Autodesk Inventor part; units mm, degrees
ref_plane "YZ Plane" through (0, 0, 0) normal (1, 0, 0) x (0, 1, 0)
ref_plane "XZ Plane" through (0, 0, 0) normal (0, 1, 0) x (-1, 0, 0)
ref_plane "XY Plane" through (0, 0, 0) normal (0, 0, 1) x (1, 0, 0)
sketch "Sketch1" plane through (0, 0, 0) normal (0, 0, 1) x (1, 0, 0)
  line L0 (-205, -150) -> (205, -150)
  line L1 (205, -150) -> (205, 150)
  line L2 (205, 150) -> (-205, 150)
  line L3 (-205, 150) -> (-205, -150)
  line L4 (-205, -150) -> (205, 150) construction
  line L5 (205, -150) -> (-205, 150) construction
  point P0 (0, 0)
  dimension "d0" = 410
  dimension "d1" = 300
extrude "Extrusion1" add sketch "Sketch1" along normal mid plane 3
sketch "Sketch5" plane through (0, 0, 1.5) normal (0, 0, 1) x (1, 0, 0)
  circle A0 centre (-30, 10) radius 2.1
  circle A1 centre (-30, -10) radius 2.1
  circle A2 centre (30, 10) radius 2.1
  circle A3 centre (30, -10) radius 2.1
  point P0 (0, 0)
hole "Hole2" at (-30, 10, 1.5) at (-30, -10, 1.5) at (30, 10, 1.5) at (30, -10, 1.5) direction (0, 0, -1) diameter 5.5 end through all countersink diameter 11 countersink angle 90
fillet "Fillet2" radius 3 4 edges at (205, -150, 0) (205, 150, 0) (-205, 150, 0) (-205, -150, 0)
properties part number "PBLMK-041-1" material "Aluminum"
Design review of the part built by this model. Coordinates are the model's own, in mm. Coordinates: 2 decimals unless noted, no trailing zeros. Put each result on its own line as item: value.
1) The part is to be moulded in two halves that separate along X. For faces 1 (the face through (-3, 2, 1.5)), 2 (the face through (33, 10, -1)), say which applies: released by +X, released by -X, zero draft, split by the parting line, or undercut.
Response values:
face 1: zero draft
face 2: undercut
2) Wall thickness on L1, parallel to Y at x = 30, z = -1.35; L2, parallel to X at y = -10, z = -1.4: over which ranges is each line inside the solid? List them lowest first. Write a range as from..to.
Response values:
L1: y = -150..-12.75, -7.25..7.25, 12.75..150
L2: x = -205..-32.75, -27.25..27.25, 32.75..205
3) Insertion check: P1, Ø5, axis at x = -30, y = -10, coming from the +Z side; P2, Ø9, axis at x = -30, y = 10, coming from the +Z side. Each pin has a flat end and moves straight along its axis. Give the tip position at first contact, or say it passes through.
Response values:
P1: passes through
P2: stops at z = 0.5
